from build123d import *

# Parameters (mm, degrees)
EXTRUDE_1_DEPTH = 60
SKETCH_1_5_R    = 10
SKETCH_1_5_R_2  = 4
SKETCH_1_5_R_3  = 4.5
EXTRUDE_2_DEPTH = 20


with BuildPart() as part:
    # Sketch 1 → Extrude 1 (new body)
    with BuildSketch(Plane.XY):
        with BuildLine():
            ThreePointArc((20, 0), (-8.94427191, -17.88854382), (-12, 16))
            Line((-12, 16), (-12, 24.186773245))
            ThreePointArc((-12, 24.186773245), (-25.34332345, 9.312140276), (-24.805215663, -10.663080039))
            ThreePointArc((-24.805215663, -10.663080039), (-19.091883092, -19.091883092), (-10.663080039, -24.805215663))
            ThreePointArc((-10.663080039, -24.805215663), (14.850872684, -22.548870937), (27, 0))
            ThreePointArc((27, 0), (22.945587811, 14.230249471), (12, 24.186773245))
            Line((12, 24.186773245), (12, 16))
            ThreePointArc((12, 16), (17.88854382, 8.94427191), (20, 0))
        make_face()
        with BuildLine():
            ThreePointArc((-12, 16), (-9.597918943, 17.546508256), (-7, 18.734993995))
            Line((-7, 18.734993995), (-7, 26.076809621))
            ThreePointArc((-7, 26.076809621), (-9.546887418, 25.255829834), (-12, 24.186773245))
            Line((-12, 24.186773245), (-12, 16))
        make_face()
        with BuildLine():
            Line((-7, 26.076809621), (-7, 18.734993995))
            ThreePointArc((-7, 18.734993995), (0, 20), (7, 18.734993995))
            Line((7, 18.734993995), (7, 26.076809621))
            ThreePointArc((7, 26.076809621), (0, 27), (-7, 26.076809621))
        make_face()
        with BuildLine():
            Line((7, 26.076809621), (7, 18.734993995))
            ThreePointArc((7, 18.734993995), (9.597918943, 17.546508256), (12, 16))
            Line((12, 16), (12, 24.186773245))
            ThreePointArc((12, 24.186773245), (9.546887418, 25.255829834), (7, 26.076809621))
        make_face()
    extrude(amount=EXTRUDE_1_DEPTH)

    # Sketch 1_5 → Extrude 2 (add)
    # profile 1 of 4: a face of its own
    with BuildSketch(Plane.XY):
        with BuildLine():
            ThreePointArc((-10.663080039, -24.805215663), (-19.091883092, -19.091883092), (-24.805215663, -10.663080039))
            Line((-24.805215663, -10.663080039), (-38.890872965, -24.748737342))
            ThreePointArc((-38.890872965, -24.748737342), (-27.99297083, -22.581009828), (-21.819805153, -31.819805153))
            ThreePointArc((-21.819805153, -31.819805153), (-22.581009828, -35.646639477), (-24.748737342, -38.890872965))
            Line((-24.748737342, -38.890872965), (-10.663080039, -24.805215663))
        make_face()
    # profile 2 of 4: a face of its own
    with BuildSketch(Plane.XY):
        with Locations((-31.819805153, -31.819805153)):
            Circle(SKETCH_1_5_R)
        with Locations((-31.819805153, -31.819805153)):
            Circle(SKETCH_1_5_R_2, mode=Mode.SUBTRACT)
    # profile 3 of 4: a face of its own
    with BuildSketch(Plane.XY):
        with BuildLine():
            ThreePointArc((-12, 24.186773245), (-9.546887418, 25.255829834), (-7, 26.076809621))
            Line((-7, 26.076809621), (-7, 40))
            ThreePointArc((-7, 40), (0, 47), (7, 40))
            Line((7, 40), (7, 26.076809621))
            ThreePointArc((7, 26.076809621), (9.546887418, 25.255829834), (12, 24.186773245))
            Line((12, 24.186773245), (12, 40))
            ThreePointArc((12, 40), (0, 52), (-12, 40))
            Line((-12, 40), (-12, 24.186773245))
        make_face()
    # profile 4 of 4: a face of its own
    with BuildSketch(Plane.XY):
        with BuildLine():
            Line((-7, 40), (-7, 26.076809621))
            ThreePointArc((-7, 26.076809621), (0, 27), (7, 26.076809621))
            Line((7, 26.076809621), (7, 40))
            ThreePointArc((7, 40), (0, 47), (-7, 40))
        make_face()
        with Locations((0, 40)):
            Circle(SKETCH_1_5_R_3, mode=Mode.SUBTRACT)
    extrude(amount=EXTRUDE_2_DEPTH)


solid = part.part
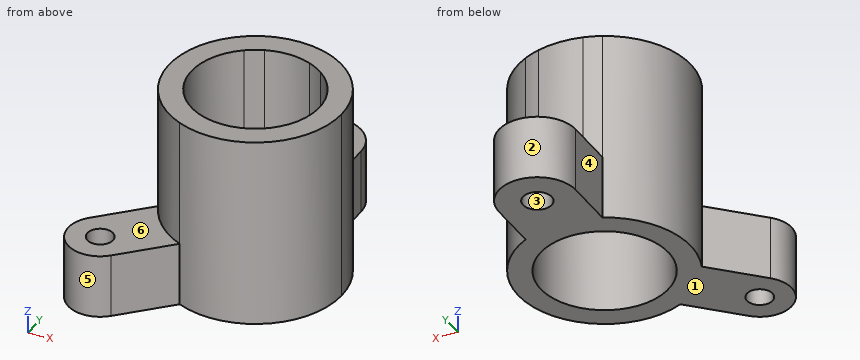
Design review of the part built by this model. Coordinates are the model's own, in mm. Face numbers are marked on the shaded views. A direction names the side the tool comes from. Round coordinates to 2 decimals unless told otherwise and drop trailing zeros. Loops run counter-clockwise (first coordinate to the right, second up) from the corner with the lowest first, then second, coordinate; pieces in that order, holes last. Notation, with made-up numbers: (55, -17) - (64, -17) arc R23 cw to (64, 5) - close; hole circle Ø4 at (78.5, 51.25). An arc over 180 degrees is marked (long way). One line per question, with ' | ' between items.
1. Draft analysis for pull direction X (two halves, no side actions). For the marked faces 1, 2, 3 and 4, state which applies: released by +X, released by -X, zero draft, split by the parting line, or undercut.
Results are:
face 1: zero draft | face 2: split by the parting line | face 3: undercut | face 4: released by -X
2. For L1, parallel to X at y = 0, z = 31.5; L2, parallel to X at y = -33, z = 11; L3, parallel to Y at x = -10.5, z = 48.5, list the stretches that pass through material, from the lowest coordinate up. Write a range as [from, to].
Results are:
L1: x = [-27, -20], [20, 27] | L2: x = [-41.75, -35.64], [-28, -18.86] | L3: y = [-24.87, -17.02], [17.02, 24.87]
3. We need section A-A, the plane x = 0. State the section outline as (y, z) points.
Results are:
outline: (-27, 0) - (-20, 0) - (-20, 60) - (-27, 60) - close; (20, 0) - (35.5, 0) - (35.5, 20) - (27, 20) - (27, 60) - (20, 60) - close; (44.5, 0) - (52, 0) - (52, 20) - (44.5, 20) - close
4. For the marked faces 5 and 6, list the 3-axis set-ups (+Z, -Z, +X, -X, +Y, -Y) from which the entire face can be reached by the end or side of a thin tool; tool diameter is ignored.
Results are:
face 5: +Z, -Z | face 6: +Z, -X, -Y
5. We need section D-D, the plane x = -16.5. State the section outline as (y, z) points.
Results are:
outline: (-30.64, 0) - (-11.3, 0) - (-11.3, 60) - (-21.37, 60) - (-21.37, 20) - (-30.64, 20) - close; (11.3, 0) - (21.37, 0) - (21.37, 60) - (11.3, 60) - close
6. We need section C-C, the plane y = 30. State the section outline as (x, z) points.
Results are:
outline: (-12, 0) - (12, 0) - (12, 20) - (-12, 20) - close
7. Clearance check with flat-ended pins moving along their axes: P1, Ø25, axis at x = -21, y = -31, coming from the +Z side; P2, Ø12.5, axis at y = 35, z = 10.5, coming from the +X side; P3, Ø6, axis at y = -11.5, z = 7, coming from the -X side; P4, Ø9, axis at x = -31.82, y = -31.82, coming from the +Z side. State where each tip first meets the part, or that it passes through.
Results are:
P1: stops at z = 60 | P2: stops at x = 12 | P3: stops at x = -28.64 | P4: stops at z = 20
8. We need section B-B, the plane x = 16. State the section outline as (y, z) points, and give its area (3 significant figures).
Results are:
outline: (-21.75, 0) - (-12, 0) - (-12, 60) - (-21.75, 60) - close; (12, 0) - (21.75, 0) - (21.75, 60) - (12, 60) - close | area: 1,170 mm²
